For this review, take the finished solid that the model builds, in its own axes (mm). Face numbers are marked on the shaded views. A direction names the side the tool comes from. Coordinates: 2 decimals unless noted, no trailing zeros. Order: outer loops, then holes, each group sorted by start corner. A loop starts at its lowest first (then second) coordinate and runs counter-clockwise, first axis right, second up. Notation, with made-up numbers: (-31, 30.25) -> (-27, 30.25) arc R25 ccw to (-27, 63.25) -> close; hole circle Ø5 at (66, 35.5). An arc over 180 degrees is marked (long way). Return JSON: item names as keys, results as strings. Group by question number.
Item 1: Insertion check: pin 1 (2.5 mm diameter, centred on x = -22.93, y = -17.75, fed in from -Z); pin 2 (4.5 mm diameter, centred on x = -28, y = 17.74, fed in from +Z); pin 3 (4 mm diameter, centred on x = -10, y = 8.5, fed in from +Z); pin 4 (0.9 mm diameter, centred on x = -28, y = 8, fed in from -Z). Each pin has a flat end and moves straight along its axis. Give the tip position at first contact, or say it passes through.
Item 2: Take a section at A-A (z = 11.75). Write out the cut boundary in (x, y).
Item 3: Take a section at B-B (y = -12.68). Count the separate pieces of the cut face and the enclosed holes in it, then the cut area to 3 significant figures.
Item 4: Machinability: for the marked faces 1 and 2, which of the approach directions +Z, -Z, +X, -X, +Y, -Y give a long, thin tool a straight path to every point of the face, cutting with its end or side? Answer none if there is none.
Item 5: Take a section at C-C (x = -10). Write out the cut boundary in (y, z).
Item 6: Draft analysis for pull direction X (two halves, no side actions). For the marked faces 3, 4 and 5, state which applies: +X half, -X half, draft (parallel to the pull), parting line (faces both ways), or undercut.
Item 7: For line 1 along X through (y, z) = (16, 16); line 2 along X through (y, z) = (-2.54, 0.8); line 3 along Y through (x, z) = (10, 8.25), list the stretches that pass through material, from the lowest coordinate up.
```python
from build123d import *

# Parameters (mm, degrees)
SKETCH002_W           = 2
SKETCH002_H           = 39.5
EXTRUDE002_DEPTH      = 9.5
SKETCH001_R           = 2.5
SKETCH001_R_2         = 1.25
SKETCH001_W           = 2
SKETCH001_H           = 39.5
EXTRUDE001_DEPTH      = 8.5
EXTRUDE001_DEPTH_BACK = 1
SKETCH005_R           = 2
EXTRUDE004_DEPTH      = 2
SKETCH_W              = 68
SKETCH_H              = 47.5
EXTRUDE_DEPTH         = 22
FILLET_R              = 6
THICKNESS_T           = -2
FILLET001_R           = 0.9
FILLET002_R           = 1.5
POCKET001_DEPTH       = 5


with BuildPart() as extrude002:
    # Sketch002 (on Face6 of Extrude001) → Extrude002 (new body)
    with BuildSketch(Plane.XY.offset(10.5)):
        with Locations((13, 0)):
            Rectangle(SKETCH002_W, SKETCH002_H)
    extrude(amount=EXTRUDE002_DEPTH)


with BuildPart() as fusion:
    # Sketch001 (on Face19 of Thickness) → Extrude001 (new body, two sides)
    with BuildSketch(Plane.XY.offset(2)) as extrude001_sk:
        with Locations((-29.5, 8.5)):
            Circle(SKETCH001_R)
        with Locations((-29.5, 8.5)):
            Circle(SKETCH001_R_2, mode=Mode.SUBTRACT)
        with Locations((-10, 8.5)):
            Circle(SKETCH001_R)
        with Locations((-10, 8.5)):
            Circle(SKETCH001_R_2, mode=Mode.SUBTRACT)
        with Locations((-29.5, -8.5)):
            Circle(SKETCH001_R)
        with Locations((-29.5, -8.5)):
            Circle(SKETCH001_R_2, mode=Mode.SUBTRACT)
        with Locations((-10, -8.5)):
            Circle(SKETCH001_R)
        with Locations((-10, -8.5)):
            Circle(SKETCH001_R_2, mode=Mode.SUBTRACT)
        with Locations((13, 0)):
            Rectangle(SKETCH001_W, SKETCH001_H)
    extrude(amount=EXTRUDE001_DEPTH)
    extrude(extrude001_sk.sketch, amount=-EXTRUDE001_DEPTH_BACK)

    # Fusion: union Extrude002
    add(extrude002.part)


with BuildPart() as extrude004:
    # Sketch005 (on Face2 of Thickness) → Extrude004 (new body)
    with BuildSketch(Plane(origin=(0, 0, 0), x_dir=(1, 0, 0), z_dir=(0, 0, -1))):
        with Locations((-28, 17.75)):
            Circle(SKETCH005_R)
        with Locations((-22.93, 17.75)):
            Circle(SKETCH005_R)
        with Locations((-17.86, 17.75)):
            Circle(SKETCH005_R)
        with Locations((-12.79, 17.75)):
            Circle(SKETCH005_R)
        with Locations((-28, 12.68)):
            Circle(SKETCH005_R)
        with Locations((-22.93, 12.68)):
            Circle(SKETCH005_R)
        with Locations((-17.86, 12.68)):
            Circle(SKETCH005_R)
        with Locations((-12.79, 12.68)):
            Circle(SKETCH005_R)
        with Locations((-28, 7.61)):
            Circle(SKETCH005_R)
        with Locations((-22.93, 7.61)):
            Circle(SKETCH005_R)
        with Locations((-17.86, 7.61)):
            Circle(SKETCH005_R)
        with Locations((-12.79, 7.61)):
            Circle(SKETCH005_R)
        with Locations((-28, 2.54)):
            Circle(SKETCH005_R)
        with Locations((-22.93, 2.54)):
            Circle(SKETCH005_R)
        with Locations((-17.86, 2.54)):
            Circle(SKETCH005_R)
        with Locations((-12.79, 2.54)):
            Circle(SKETCH005_R)
        with Locations((-28, -2.53)):
            Circle(SKETCH005_R)
        with Locations((-22.93, -2.53)):
            Circle(SKETCH005_R)
        with Locations((-17.86, -2.53)):
            Circle(SKETCH005_R)
        with Locations((-12.79, -2.53)):
            Circle(SKETCH005_R)
        with Locations((-28, -7.6)):
            Circle(SKETCH005_R)
        with Locations((-22.93, -7.6)):
            Circle(SKETCH005_R)
        with Locations((-17.86, -7.6)):
            Circle(SKETCH005_R)
        with Locations((-12.79, -7.6)):
            Circle(SKETCH005_R)
        with Locations((-28, -12.67)):
            Circle(SKETCH005_R)
        with Locations((-22.93, -12.67)):
            Circle(SKETCH005_R)
        with Locations((-17.86, -12.67)):
            Circle(SKETCH005_R)
        with Locations((-12.79, -12.67)):
            Circle(SKETCH005_R)
        with Locations((-28, -17.74)):
            Circle(SKETCH005_R)
        with Locations((-22.93, -17.74)):
            Circle(SKETCH005_R)
        with Locations((-17.86, -17.74)):
            Circle(SKETCH005_R)
        with Locations((-12.79, -17.74)):
            Circle(SKETCH005_R)
    extrude(amount=-EXTRUDE004_DEPTH)


with BuildPart() as body003:
    # Sketch → Extrude (new body)
    with BuildSketch(Plane.XY):
        Rectangle(SKETCH_W, SKETCH_H)
    extrude(amount=EXTRUDE_DEPTH)

    # Fillet
    fillet_edges = [body003.edges().sort_by_distance(p)[0] for p in [
        (-34, 23.75, 11),
        (34, 23.75, 11),
        (34, -23.75, 11),
        (-34, -23.75, 11),
    ]]
    fillet(fillet_edges, radius=FILLET_R)

    # Thickness
    thickness_openings = [body003.faces().sort_by_distance(p)[0] for p in [
        (0, 0, 22),
    ]]
    offset(amount=THICKNESS_T, openings=thickness_openings)

    # Cut: cut Extrude004
    add(extrude004.part, mode=Mode.SUBTRACT)

    # Fusion001: union Fusion
    add(fusion.part)

    # Fillet001
    fillet001_edges = [body003.edges().sort_by_distance(p)[0] for p in [
        (14, 19.75, 6.25),
        (12, 19.75, 6.25),
        (12, -19.75, 6.25),
        (14, -19.75, 6.25),
        (12, 19.75, 15.25),
        (14, 19.75, 15.25),
        (12, -19.75, 15.25),
        (14, -19.75, 15.25),
    ]]
    fillet(fillet001_edges, radius=FILLET001_R)

    # Fillet002
    fillet002_edges = [body003.edges().sort_by_distance(p)[0] for p in [
        (13.736396, 19.486396, 2),
        (14, 0, 2),
        (13.736396, -19.486396, 2),
        (13, -19.75, 2),
        (12.263604, -19.486396, 2),
        (12, 0, 2),
        (12.263604, 19.486396, 2),
    ]]
    fillet(fillet002_edges, radius=FILLET002_R)

    # Sketch006 (on Face92 of Fillet002) → Pocket001 (cut)
    with BuildSketch(Plane(origin=(0, 23.75, 0), x_dir=(-1, 0, 0), z_dir=(0, 1, 0))):
        with BuildLine():
            ThreePointArc((-25.5, 10), (-29, 6.5), (-25.5, 3))
            Line((-25.5, 3), (-20.5, 3))
            ThreePointArc((-20.5, 3), (-17, 6.5), (-20.5, 10))
            Line((-20.5, 10), (-25.5, 10))
        make_face()
    extrude(amount=-POCKET001_DEPTH, mode=Mode.SUBTRACT)


solid = body003.part
```
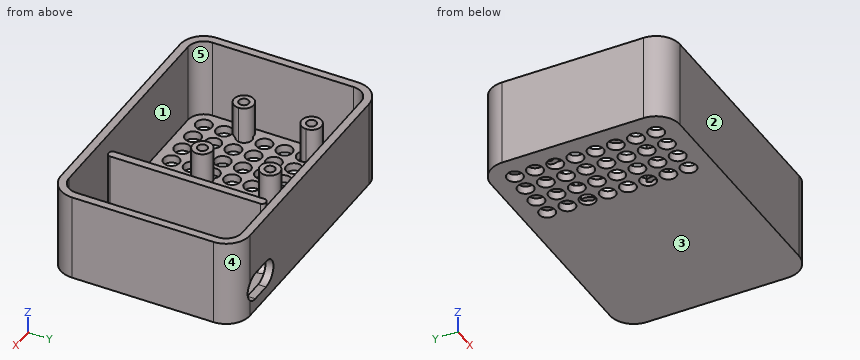
Findings below:
{
 "1": {"pin 1": "passes through", "pin 2": "stops at z = 2", "pin 3": "stops at z = 10.5", "pin 4": "stops at z = 1"},
 "2": {"outline": "(-34, -17.75) arc R6 ccw to (-28, -23.75) -> (28, -23.75) arc R6 ccw to (34, -17.75) -> (34, 17.75) arc R6 ccw to (28, 23.75) -> (-28, 23.75) arc R6 ccw to (-34, 17.75) -> close; (12, -18.85) arc R0.9 ccw to (12.9, -19.75) -> (13.1, -19.75) arc R0.9 ccw to (14, -18.85) -> (14, 18.85) arc R0.9 ccw to (13.1, 19.75) -> (12.9, 19.75) arc R0.9 ccw to (12, 18.85) -> close; hole (-32, -17.75) arc R4 ccw to (-28, -21.75) -> (28, -21.75) arc R4 ccw to (32, -17.75) -> (32, 17.75) arc R4 ccw to (28, 21.75) -> (-28, 21.75) arc R4 ccw to (-32, 17.75) -> close"},
 "3": {"separate pieces": "5", "enclosed holes": "0", "area": "221 mm2"},
 "4": {"face 1": "+Z", "face 2": "+Z, -Z, +X, -X, -Y"},
 "5": {"outline": "(-23.75, 0) -> (23.75, 0) -> (23.75, 22) -> (21.75, 22) -> (21.75, 2) -> (11, 2) -> (11, 10.5) -> (9.75, 10.5) -> (9.75, 2) -> (7.25, 2) -> (7.25, 10.5) -> (6, 10.5) -> (6, 2) -> (-6, 2) -> (-6, 10.5) -> (-7.25, 10.5) -> (-7.25, 2) -> (-9.75, 2) -> (-9.75, 10.5) -> (-11, 10.5) -> (-11, 2) -> (-21.75, 2) -> (-21.75, 22) -> (-23.75, 22) -> close"},
 "6": {"face 3": "draft", "face 4": "+X half", "face 5": "undercut"},
 "7": {"line 1": "x = -34 to -32, 12 to 14, 32 to 34", "line 2": "x = -34 to -30, -26 to -24.93, -20.93 to -19.86, -15.86 to -14.79, -10.79 to 34", "line 3": "y = -23.75 to -21.75, 21.75 to 23.75"}
}
